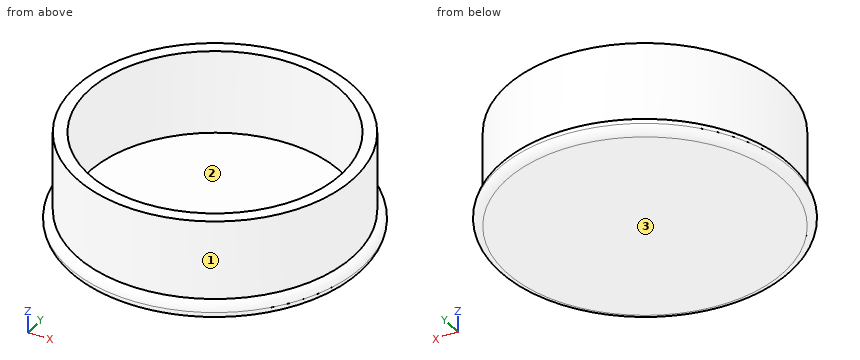
```python
from build123d import *

# Parameters (mm, degrees)
TORUS_R           = 1
CYLINDER_R        = 15.1
CYLINDER_DEPTH    = 12.5
CYLINDER001_R     = 16.6
CYLINDER001_DEPTH = 11.5


with BuildPart() as lip:
    # Torus → Torus (revolve)
    with BuildSketch(Plane(origin=(0, 0, -0.5), x_dir=(1, 0, 0), z_dir=(0, -1, 0))):
        with Locations((16.6, 0)):
            Circle(TORUS_R)
    revolve(axis=Axis((0, 0, -0.5), (0, 0, 1)))


with BuildPart() as internal:
    # Cylinder → Cylinder (new body)
    with BuildSketch(Plane.XY):
        Circle(CYLINDER_R)
    extrude(amount=CYLINDER_DEPTH)


with BuildPart() as fusion:
    # Cylinder001 → Cylinder001 (new body)
    with BuildSketch(Plane.XY.offset(-1.5)):
        Circle(CYLINDER001_R)
    extrude(amount=CYLINDER001_DEPTH)

    # Cut: cut Internal
    add(internal.part, mode=Mode.SUBTRACT)

    # Fusion: union Lip
    add(lip.part)


solid = fusion.part
```
CAD build for the part. Positions are in the model's coordinates, mm. Face numbers are marked on the shaded views. Round coordinates to 2 decimals unless told otherwise and drop trailing zeros. Order: outer loops, then holes, each group sorted by start corner. A loop starts at its lowest first (then second) coordinate and runs counter-clockwise, first axis right, second up. Notation, with made-up numbers: (6.25, -1.5) - (59.25, -1.5) arc R10 ccw to (59.25, 14.5) - close; hole circle Ø8 at (82.5, 65). An arc over 180 degrees is marked (long way). Answer in a Markdown table with one row per item. Add a question column.
(1) Band-saw the part on C-C on z = 3.75. List the corners of the cut face in (x, y), and give its area (3 significant figures).
(2) Mould opens along X. For the marked faces 1, 2 and 3 say: +X half, -X half, draft (parallel to the pull), parting line (faces both ways), or undercut.
(3) Band-saw the part on A-A on x = 0. List the corners of the cut face in (y, z).
(4) Probe L1, parallel to Y at x = 0, z = 5.5; L2, parallel to X at y = 12, z = 2.75; L3, parallel to X at y = -3.5, z = 7.75. List the from-to ranges inside material, lowest first. Write a range as [from, to].
(5) Drop flat-ended pins along their axis: pin 1 Ø1 at (x, y) = (2, -1) entering from +Z; pin 2 Ø5 at (y, z) = (11, 3.5) entering from +X. Give the stop position or say it passes through.
Data:
| question | item | result |
|---|---|---|
| 1 | outline | circle Ø33.2 at (0, 0); hole circle Ø30.2 at (0, 0) |
| 1 | area | 149 mm^2 |
| 2 | face 1 | parting line |
| 2 | face 2 | undercut |
| 2 | face 3 | draft |
| 3 | outline | (-16.6, -1.5) - (16.6, -1.5) arc R1 ccw to (16.6, 0.5) - (16.6, 10) - (15.1, 10) - (15.1, 0) - (-15.1, 0) - (-15.1, 10) - (-16.6, 10) - (-16.6, 0.5) arc R1 ccw to start |
| 4 | L1 | y = [-16.6, -15.1], [15.1, 16.6] |
| 4 | L2 | x = [-11.47, -9.17], [9.17, 11.47] |
| 4 | L3 | x = [-16.23, -14.69], [14.69, 16.23] |
| 5 | pin 1 | stops at z = 0 |
| 5 | pin 2 | stops at x = 14.26 |
